Geometry: final body of the model. Coordinates: model frame, mm. Face numbers are marked on the shaded views. A direction names the side the tool comes from. Round coordinates to 2 decimals unless told otherwise and drop trailing zeros. Loops run counter-clockwise (first coordinate to the right, second up) from the corner with the lowest first, then second, coordinate; pieces in that order, holes last. Notation, with made-up numbers: M -33,39.25 L -27,39.25 A23 ccw -27,65.25 Z; hole C -11,15.5 d11. An arc over 180 degrees is marked long. Answer as a JSON object with one key per item and string values.
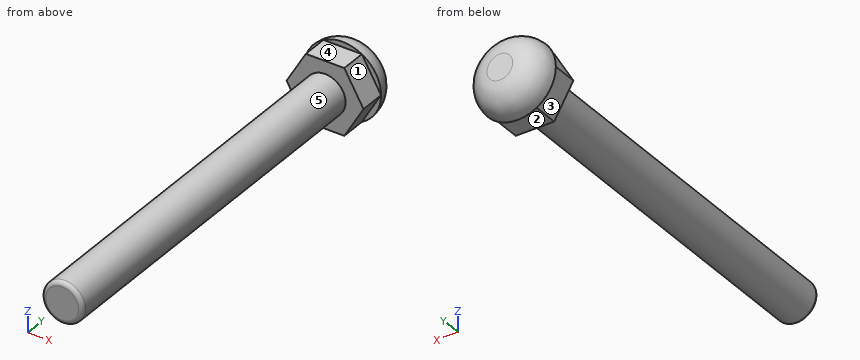
Autodesk Inventor part; units mm, degrees
ref_plane "YZ Plane" through (0, 0, 0) normal (1, 0, 0) x (0, 1, 0)
ref_plane "XZ Plane" through (0, 0, 0) normal (0, 1, 0) x (-1, 0, 0)
ref_plane "XY Plane" through (0, 0, 0) normal (0, 0, 1) x (1, 0, 0)
sketch "Sketch1" plane through (0, 0, 0) normal (0, 1, 0) x (-1, 0, 0)
  circle A0 centre (0, 0) radius 4.7625
  dimension "d0" = 9.525
extrude "Extrusion1" add sketch "Sketch1" along normal blind 3.175
fillet "Fillet1" radius 3.175 1 edges at (4.7625, 3.175, 0)
sketch "Sketch2" plane through (0, 0, 0) normal (0, -1, 0) x (1, 0, 0)
  circle A0 centre (0, 0) radius 2.54
  dimension "d4" = 5.08
extrude "Extrusion2" add sketch "Sketch2" along normal blind 50.8
fillet "Fillet2" radius 0.508 1 edges at (-2.54, -50.8, 0)
thread "Thread1"
sketch "Sketch3" plane through (0, 0, 0) normal (0, -1, 0) x (1, 0, 0)
  circle A0 centre (0, 0) radius 1.5875
  circle A1 centre (0, 0) radius 4.7625
  line L0 (-4.7625, 0) -> (-2.3813, 4.1244)
  line L1 (-2.3813, 4.1244) -> (2.3812, 4.1244)
  line L2 (2.3812, 4.1244) -> (4.7625, 0)
  line L3 (4.7625, 0) -> (2.3813, -4.1244)
  line L4 (2.3813, -4.1244) -> (-2.3812, -4.1244)
  line L5 (-2.3812, -4.1244) -> (-4.7625, 0)
extrude "Extrusion3" add sketch "Sketch3" along normal blind 3.175 contours L3 L4 L5 L0 L1 L2
properties part number "2in Bolt w Nut"
1) First-contact query: pin 1 (1.5 mm diameter, centred on y = -4.5, z = 1, fed in from -X); pin 2 (1.5 mm diameter, centred on y = -17, z = -0.5, fed in from +X); pin 3 (3 mm diameter, centred on x = 1, y = -38.5, fed in from -Z). Flat tips, straight axial feed; report the tip coordinate or a pass-through.
Geometry results:
{"pin 1": "x = -2.53", "pin 2": "x = 2.54", "pin 3": "z = -2.54"}
2) Line query: probe 1 along Z at (x, y) = (1.5, -1.5); probe 2 along X at (y, z) = (-46, -0.5); probe 3 along Y at (x, z) = (1.5, 2.25) (3 decimals). Output: solid intervals per line, ascending.
Geometry results:
{"probe 1": "-4.12 to 4.12", "probe 2": "-2.49 to 2.49", "probe 3": "-3.175 to 2.972"}
3) Set-up query: the marked faces 1, 2, 3, 4 and 5. Return all of +Z, -Z, +X, -X, +Y, -Y with unobstructed straight access to the full face (end or side cutting, diameter ignored); none if empty.
Geometry results:
{"face 1": "+Z, +X, -Y", "face 2": "-Z, +X, -X, -Y", "face 3": "-Z, -X, -Y", "face 4": "+Z, +X, -X, -Y", "face 5": "-Y"}
4) Cut plane A-A on y = -27.5. Return the cut outline in (x, z).
Geometry results:
{"outline": "C 0,0 d5.08"}
